Geometry: final body of the model. Coordinates: model frame, mm. Face numbers are marked on the shaded views. A direction names the side the tool comes from. Give positions to 0.01 mm unless a question says otherwise; leave off trailing zeros. Write each loop counter-clockwise with the first axis right and the second up, starting at its lowest first coordinate (ties: lowest second). Pieces come first, ordered by that corner, then holes. Notation, with made-up numbers: (81, 80.25) -> (94, 80.25) arc R24 cw to (94, 106.25) -> close; hole circle Ø1 at (-12.5, -15). An arc over 180 degrees is marked (long way). Answer in a Markdown table with one row per item. Add a question column.
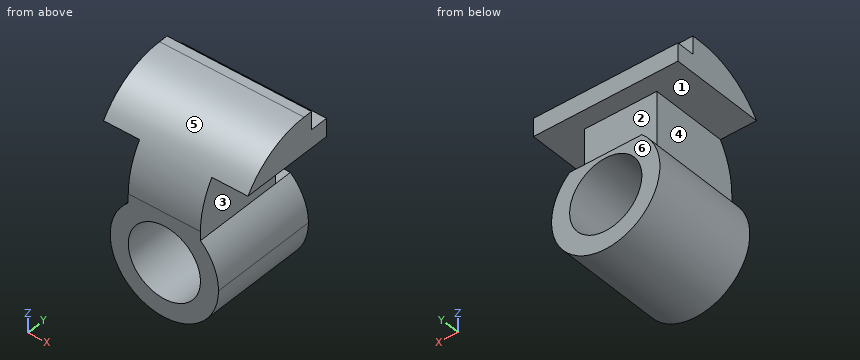
from build123d import *

# Parameters (mm, degrees)
F0_R     = 25.4
F1_DEPTH = 76.2
F2_W     = 12.7
F2_H     = 12.7
F3_DEPTH = 101.601
F4_R     = 57.15
F5_W     = 12.7
F5_H     = 38.0991366858
F6_DEPTH = 76.201


with BuildPart() as f1:
    # F0 (on Front) → F1 (new body)
    with BuildSketch(Plane.XZ):
        with BuildLine():
            Line((50.8, -12.7), (50.8, 12.7))
            Line((50.8, 12.7), (-50.8, 12.7))
            Line((-50.8, 12.7), (-50.8, -12.7))
            Line((-50.8, -12.7), (-25.4, -12.7))
            Line((-25.4, -12.7), (-25.4, -50.7991366858))
            ThreePointArc((-25.4, -50.7991366858), (0, -41.0972), (25.4, -50.7991366858))
            Line((25.4, -50.7991366858), (25.4, -12.7))
            Line((25.4, -12.7), (50.8, -12.7))
        make_face()
        with BuildLine():
            ThreePointArc((38.1, -79.1972), (34.7803824016, -63.6429401333), (25.4, -50.7991366858))
            ThreePointArc((25.4, -50.7991366858), (0, -41.0972), (-25.4, -50.7991366858))
            ThreePointArc((-25.4, -50.7991366858), (-15.5542598667, -113.9775824016), (38.1, -79.1972))
        make_face()
        with Locations((0, -79.1972)):
            Circle(F0_R, mode=Mode.SUBTRACT)
    extrude(amount=F1_DEPTH)

    # F2 (on face) → F3 (cut, through all)
    with BuildSketch(Plane(origin=(-50.8, 0, 0), x_dir=(0, -1, 0), z_dir=(-1, 0, 0))):
        with Locations((6.35, 6.35)):
            Rectangle(F2_W, F2_H)
    extrude(amount=-F3_DEPTH, mode=Mode.SUBTRACT)

    # F4
    f4_edges = [f1.edges().sort_by_distance(p)[0] for p in [
        (0, -76.2, 12.7),
    ]]
    fillet(f4_edges, radius=F4_R)

    # F5 (on face) → F6 (cut, through all)
    with BuildSketch(Plane(origin=(-25.4, 0, 0), x_dir=(0, -1, 0), z_dir=(-1, 0, 0))):
        with Locations((6.35, -31.7495683429)):
            Rectangle(F5_W, F5_H)
    extrude(amount=-F6_DEPTH, mode=Mode.SUBTRACT)


solid = f1.part
Q1. Section C-C on z = -93.5. Return loops of the section in (x, y), and give its area (3 significant figures).
Q2. Section A-A on y = -6.5. Return loops of the section in (x, z).
Q3. Pull-direction query (Z, two-part tool) for the marked faces 4, 5 and 6; classes: +Z half, -Z half, draft (parallel to the pull), parting line (faces both ways), or undercut.
Q4. Section D-D on x = 44. Return loops of the section in (y, z), and give its area (3 significant figures).
Q5. Line query: probe 1 along X at (y, z) = (-37.5, -29.5); probe 2 along X at (y, z) = (-3.5, -99.5); probe 3 along X at (y, z) = (-71, -76.5). Output: solid intervals per line, ascending. Write a range as from..to.
Q6. Access query for the marked faces 1, 2 and 3. Directions: +Z, -Z, +X, -X, +Y, -Y. A direction counts if a zero-diameter tool reaches every point of the face in a straight line with its end or side. Return the directions, or none.
Q7. Contact query for flat-ended pins moving along their axis: pin 1 Ø6.5 at (x, y) = (18, -4) entering from +Z; pin 2 Ø3 at (y, z) = (-29, -36) entering from +X; pin 3 Ø10 at (x, z) = (-9, 9) entering from +Y. Output: stop coordinate, or through.
Q8. Section B-B on x = 0. Return loops of the section in (y, z).
Checks:
| question | item | result |
|---|---|---|
| 1 | outline | (-35.31, -76.2) -> (-20.99, -76.2) -> (-20.99, 0) -> (-35.31, 0) -> close; (20.99, -76.2) -> (35.31, -76.2) -> (35.31, 0) -> (20.99, 0) -> close |
| 1 | area | 2,180 mm^2 |
| 2 | outline | (-50.8, -12.7) -> (50.8, -12.7) -> (50.8, 0) -> (-50.8, 0) -> close; (-25.4, -50.8) arc R38.1 ccw (long way) to (25.4, -50.8) -> close; hole circle Ø50.8 at (0, -79.2) |
| 3 | face 4 | undercut |
| 3 | face 5 | +Z half |
| 3 | face 6 | draft |
| 4 | outline | (-66.57, -12.7) -> (0, -12.7) -> (0, 0) -> (-12.7, 0) -> (-12.7, 12.7) -> (-19.05, 12.7) arc R57.15 ccw to start |
| 4 | area | 1,170 mm^2 |
| 5 | probe 1 | -25.4..25.4 |
| 5 | probe 2 | -32.24..-15.26, 15.26..32.24 |
| 5 | probe 3 | -38..-25.26, 25.26..38 |
| 6 | face 1 | +Y |
| 6 | face 2 | +X, -X, +Y |
| 6 | face 3 | +X, +Y, -Y |
| 7 | pin 1 | z = 0 |
| 7 | pin 2 | x = 25.4 |
| 7 | pin 3 | y = -12.7 |
| 8 | outline | (-76.2, -117.3) -> (0, -117.3) -> (0, -104.6) -> (-76.2, -104.6) -> close; (-76.2, -53.8) -> (0, -53.8) -> (0, -50.8) -> (-12.7, -50.8) -> (-12.7, -12.7) -> (0, -12.7) -> (0, 0) -> (-12.7, 0) -> (-12.7, 12.7) -> (-19.05, 12.7) arc R57.15 ccw to (-76.2, -44.45) -> close |
